Build history of the part. All positions in model axes, mm. A direction names the side the tool comes from. Round coordinates to 2 decimals unless told otherwise and drop trailing zeros. Write each loop counter-clockwise with the first axis right and the second up, starting at its lowest first coordinate (ties: lowest second). Pieces come first, ordered by that corner, then holes. Notation, with made-up numbers: (-0.75, 44) -> (28.25, 44) arc R15 cw to (28.25, 55) -> close; hole circle Ø1 at (50, 82.5). An arc over 180 degrees is marked (long way). Return JSON: item names as keys, results as strings.
from build123d import *

# Parameters (mm, degrees)
PAD_DEPTH   = 20
FILLET_R    = 2
FILLET001_R = 1.49
FILLET002_R = 1
FILLET003_R = 1


with BuildPart() as part:
    # Sketch → Pad (new body)
    with BuildSketch(Plane.XZ):
        Polygon((0, 15), (-3, 15), (-3, 0), (93.75, -15), (93.75, 0), (97, 0), (97, -6.5), (106.5, -6.5), (106.5, -3.5), (100, -3.5), (100, 0), (106.5, 0), (106.5, 3), (0, 3), align=None)
        Polygon((37.15, -2), (88.75, -2), (88.75, -10), align=None, mode=Mode.SUBTRACT)
    extrude(amount=PAD_DEPTH)

    # Fillet
    fillet_edges = [part.edges().sort_by_distance(p)[0] for p in [
        (-3, -10, 0),
        (93.75, -10, -15),
    ]]
    fillet(fillet_edges, radius=FILLET_R)

    # Fillet001
    fillet001_edges = [part.edges().sort_by_distance(p)[0] for p in [
        (0, -10, 15),
        (-3, -10, 15),
        (-1.5, 0, 15),
        (-1.5, -20, 15),
    ]]
    fillet(fillet001_edges, radius=FILLET001_R)

    # Fillet002
    fillet002_edges = [part.edges().sort_by_distance(p)[0] for p in [
        (37.15, -10, -2),
        (88.75, -10, -2),
        (88.75, -10, -10),
    ]]
    fillet(fillet002_edges, radius=FILLET002_R)

    # Fillet003
    fillet003_edges = [part.edges().sort_by_distance(p)[0] for p in [
        (0, -10, 3),
    ]]
    fillet(fillet003_edges, radius=FILLET003_R)


solid = part.part
Q1. Saw through at D-D on x = 23.5. List the corners of the cut face in (y, z).
Verdict:
{"outline": "(-20, -4.11) -> (0, -4.11) -> (0, 3) -> (-20, 3) -> close"}
Q2. Pin check, flat tips, straight feed: pin 1 Ø7.5 at (x, y) = (101.5, -10) entering from -Z; pin 2 Ø5 at (y, z) = (-8.5, 8.5) entering from +X; pin 3 Ø7 at (x, y) = (102, -14.5) entering from +Z. Stop position of each tip, or through.
Verdict:
{"pin 1": "stops at z = -6.5", "pin 2": "stops at x = 0", "pin 3": "stops at z = 3"}
Q3. Two-plate mould, pull along Z, no slides. Class faces 1 (the flat face through (44.42, -9.86, -7.35)), 2 (the flat face through (55.6, -20, -1.6)), 3 (the flat face through (88.75, -10, -6)): +Z half, -Z half, draft (parallel to the pull), parting line (faces both ways), or undercut.
Verdict:
{"face 1": "-Z half", "face 2": "draft", "face 3": "undercut"}
Q4. Wall check: L1, parallel to X at y = -7.5, z = 4.5; L2, parallel to Z at x = 6.5, y = -7.5; L3, parallel to Z at x = 51, y = -14. Give the ranges that are in metal, low to high.
Verdict:
{"L1": "x = -3 to 0", "L2": "z = -1.47 to 3", "L3": "z = -8.37 to -4.15, -2 to 3"}
Q5. Saw through at B-B on x = 84. List the corners of the cut face in (y, z).
Verdict:
{"outline": "(-20, -13.49) -> (0, -13.49) -> (0, -9.26) -> (-20, -9.26) -> close; (-20, -2) -> (0, -2) -> (0, 3) -> (-20, 3) -> close"}
Q6. Saw through at C-C on z = 10. List the corners of the cut face in (x, y), then the cut area to 3 significant figures.
Verdict:
{"outline": "(-3, -20) -> (0, -20) -> (0, 0) -> (-3, 0) -> close", "area": "60.0 mm²"}
Q7. 3-axis set-ups, long thin cutter, end or side, ignore diameter. For faces 4 (the flat face through (102, -10, -6.5)), 5 (the flat face through (69.049, -9.86, -6.946)), 6 (the flat face through (93.75, -10, -6)): which of +Z, -Z, +X, -X, +Y, -Y reach the whole face in a straight line?
Verdict:
{"face 4": "-Z, +X, +Y, -Y", "face 5": "+Y, -Y", "face 6": "-Z, +Y, -Y"}
